from build123d import *

# Parameters (mm, degrees)
F0_W     = 81.915
F0_H     = 81.915
F1_DEPTH = 174.625
F3_DEPTH = 174.626
F5_DEPTH = 174.626
F7_DEPTH = 174.626
F9_DEPTH = 174.626
F10_R    = 1.27
F11_R    = 1.778
F12_R    = 3.429


with BuildPart() as f1:
    # F0 (on Front) → F1 (new body)
    with BuildSketch(Plane.XZ):
        Rectangle(F0_W, F0_H)
    extrude(amount=F1_DEPTH)

    # F2 (on face) → F3 (cut, through all)
    with BuildSketch(Plane.XZ.offset(174.625)):
        Polygon((7.9375, 40.9575), (-7.9375, 40.9575), (0, 33.02), align=None)
    extrude(amount=-F3_DEPTH, mode=Mode.SUBTRACT)

    # F4 (on face) → F5 (cut, through all)
    with BuildSketch(Plane.XZ.offset(174.625)):
        Polygon((0, -25.0825), (-15.875, -40.9575), (15.875, -40.9575), align=None)
    extrude(amount=-F5_DEPTH, mode=Mode.SUBTRACT)

    # F6 (on face) → F7 (cut, through all)
    with BuildSketch(Plane.XZ.offset(174.625)):
        Polygon((-2.8575, 0), (-40.9575, 38.1), (-40.9575, -38.1), align=None)
    extrude(amount=-F7_DEPTH, mode=Mode.SUBTRACT)

    # F8 (on face) → F9 (cut, through all)
    with BuildSketch(Plane.XZ.offset(174.625)):
        Polygon((40.9575, -23.8125), (40.9575, 23.8125), (17.145, 0), align=None)
    extrude(amount=-F9_DEPTH, mode=Mode.SUBTRACT)

    # F10
    f10_edges = [f1.edges().sort_by_distance(p)[0] for p in [
        (-7.9375, -87.3125, 40.9575),
        (7.9375, -87.3125, 40.9575),
        (40.9575, -87.3125, 40.9575),
        (40.9575, -87.3125, 23.8125),
        (40.9575, -87.3125, -23.8125),
        (40.9575, -87.3125, -40.9575),
        (15.875, -87.3125, -40.9575),
        (-15.875, -87.3125, -40.9575),
        (-40.9575, -87.3125, -40.9575),
        (-40.9575, -87.3125, -38.1),
        (-40.9575, -87.3125, 38.1),
        (-40.9575, -87.3125, 40.9575),
    ]]
    fillet(f10_edges, radius=F10_R)

    # F11
    f11_edges = [f1.edges().sort_by_distance(p)[0] for p in [
        (0, -87.3125, 33.02),
    ]]
    fillet(f11_edges, radius=F11_R)

    # F12
    f12_edges = [f1.edges().sort_by_distance(p)[0] for p in [
        (0, -87.3125, -25.0825),
        (17.145, -87.3125, 0),
        (-2.8575, -87.3125, 0),
    ]]
    fillet(f12_edges, radius=F12_R)


solid = f1.part
Verification items for the finished model (mm, model axes). A direction names the side the tool comes from. Give positions to 0.01 mm unless a question says otherwise; leave off trailing zeros. Order: outer loops, then holes, each group sorted by start corner. A loop starts at its lowest first (then second) coordinate and runs counter-clockwise, first axis right, second up. Notation, with made-up numbers: M 1.25,89 L 29.25,89 A28 cw 29.25,119 Z; hole C 0,88 d1. An arc over 180 degrees is marked long. Answer as a JSON object with one key per item and string values. Group by question number.
1) Cross-section at A-A (x = -33.5). Enter the section's corners in (y, z) (1 decimal), then the cut area to 3 significant figures.
2) Scan lines: line 1 along Z through (x, y) = (-34, -28); line 2 along Z through (x, y) = (-17, -55.5); line 3 along X through (y, z) = (-27.5, -38). Record each from-to range of solid material in increasing order. Write a range as [from, to].
3) Mould release check, pull along X, two halves, no side actions. Record for faces 5 (the face through (-0.038, -86.09, -26.503)), 6 (the face through (-23.18, -88.53, -20.32)), 7 (the face through (18.566, -86.09, 0.038)), 8 (the face through (9, -174.625, 1)): released by +X, released by -X, zero draft, split by the parting line, or undercut.
4) Depth check by flat-ended pin: pin 1 Ø3 at (y, z) = (-98, 6.5) entering from +X (3 decimals); pin 2 Ø8 at (y, z) = (-143, 10.5) entering from +X (3 decimals); pin 3 Ø4 at (x, y) = (6.5, -129.5) entering from -Z. Enter the tip coordinate at first touch or a pass-through.
5) Access from +Z, -Z, +X, -X, +Y, -Y to the whole of each face (thin tool, end or side, straight path). Record for faces 1 (the face through (30.225, -88.535, 13.08)), 2 (the face through (9.06, -88.53, -34.14)), 3 (the face through (-22.69, -88.53, 19.83)), 4 (the face through (4.37, -88.53, 37.39)).
6) Cross-section at D-D (z = 20). Enter the section's corners in (x, y) (1 decimal), then the cut area to 3 significant figures.
7) Cross-section at C-C (x = 26). Enter the section's corners in (y, z) (1 decimal).
Result sheet:
{
 "1": {"outline": "M -174.6,-41 L 0,-41 L 0,-30.6 L -174.6,-30.6 Z; M -174.6,30.6 L 0,30.6 L 0,41 L -174.6,41 Z", "area": "3,600 mm2"},
 "2": {"line 1": "z = [-40.96, -31.14], [31.14, 40.96]", "line 2": "z = [-40.96, -14.14], [14.14, 40.96]", "line 3": "x = [-40.79, -12.92], [12.92, 40.96]"},
 "3": {"face 5": "undercut", "face 6": "released by -X", "face 7": "released by +X", "face 8": "zero draft"},
 "4": {"pin 1": "stops at x = 25.145", "pin 2": "stops at x = 31.645", "pin 3": "stops at z = -33.58"},
 "5": {"face 1": "+X, +Y, -Y", "face 2": "-Z, +Y, -Y", "face 3": "-X, +Y, -Y", "face 4": "+Z, +Y, -Y"},
 "6": {"outline": "M -22.9,-174.6 L 37.1,-174.6 L 37.1,0 L -22.9,0 Z", "area": "10,500 mm2"},
 "7": {"outline": "M -174.6,-41 L 0,-41 L 0,-8.9 L -174.6,-8.9 Z; M -174.6,8.9 L 0,8.9 L 0,41 L -174.6,41 Z"}
}
